Source: CAD feature listing. Evaluate the final solid. Frame: model axes, mm. Face numbers are marked on the shaded views. Coordinates: 2 decimals unless noted, no trailing zeros. Order: outer loops, then holes, each group sorted by start corner. A loop starts at its lowest first (then second) coordinate and runs counter-clockwise, first axis right, second up. Notation, with made-up numbers: (35, 71) -> (71, 71) arc R33 ccw to (71, 109) -> close; hole circle Ø10 at (84.25, -11.5). An arc over 180 degrees is marked (long way). Write item = value, one per line. Start each with the question number.
Item 1: Mould query, pull axis Z, two halves, no side actions, for the marked faces 1, 2 and 3. Classes: released by +Z, released by -Z, zero draft, split by the parting line, or undercut.
Item 2: Contact query for a flat-ended pin moving along its axis: pin 1 (1.9 mm diameter, centred on y = 6.35, z = 0, fed in from +X). Output: stop coordinate, or through.
Item 3: Section query A-A (x = -4). Count the separate pieces of the cut face and the enclosed holes in it, then the cut area to 3 significant figures.
Item 4: Section query B-B (y = 19.05). Output: boundary loops of the cut face in (x, z).
Item 5: Ray query, line 1 along Z through (x, y) = (-5.5, 19.05); line 2 along Y through (x, z) = (-1.25, 2.75) (3 decimals); line 3 along Y through (x, z) = (-8.25, -1) (3 decimals). Return the intervals inside material, ascending. Write a range as [from, to].
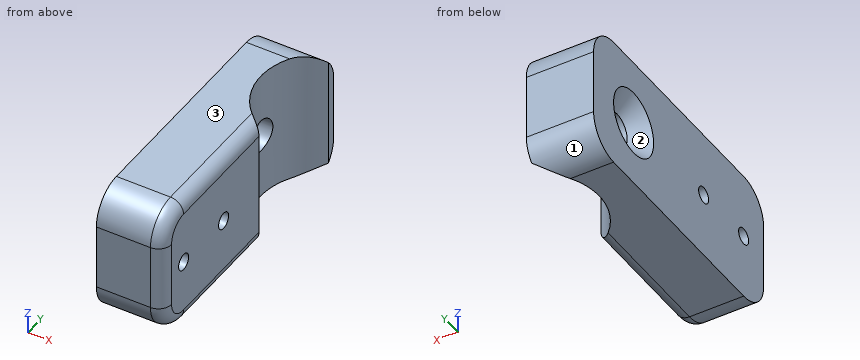
```python
from build123d import *

# Parameters (mm, degrees)
F0_R        = 1.5875
F0_R_2      = 3.175
F1_DEPTH    = 13
F3_DEPTH    = 37.5
F4_T1_DEPTH = 44.75
F5_R        = 2.54
F6_SIZE     = 3.175


# Not quite as in the source:
# - a fillet or chamfer that OpenCascade refuses, or shapes differently, is made with other operations: its cross-section is extruded or revolved along the edge and cut away or added
# - a feature names something its author has since deleted; it is built from what else it names


with BuildPart() as f1:
    # F0 (on Right) → F1 (new body)
    with BuildSketch(Plane.YZ):
        Polygon((0, 0), (0, -12.7), (53.975, -12.7), (53.975, 12.7), (0, 12.7), align=None)
        with Locations((6.35, 0)):
            Circle(F0_R, mode=Mode.SUBTRACT)
        with Locations((19.05, 0)):
            Circle(F0_R, mode=Mode.SUBTRACT)
        with Locations((41.275, 0)):
            Circle(F0_R_2, mode=Mode.SUBTRACT)
    extrude(amount=-F1_DEPTH)

    # F2 (on Top) → F3 (cut, symmetric)
    with BuildSketch(Plane.XY):
        with BuildLine():
            Line((0, 30.2764773719), (0, 52.2735226281))
            ThreePointArc((0, 52.2735226281), (-6.35, 41.275), (0, 30.2764773719))
        make_face()
    extrude(amount=F3_DEPTH, both=True, mode=Mode.SUBTRACT)

    # F4: fillet of radius 6.35 on 4 edges, made by hand

    # F4_s2 → F4_t1 (cut)
    with BuildSketch(Plane.YZ.offset(-28.875)):
        with BuildLine():
            ThreePointArc((0, -6.35), (1.8598719395, -10.8401280605), (6.35, -12.7))
            Line((6.35, -12.7), (0, -12.7))
            Line((0, -12.7), (0, -6.35))
        make_face()
        with BuildLine():
            ThreePointArc((0, 6.35), (1.8598719395, 10.8401280605), (6.35, 12.7))
            Line((6.35, 12.7), (0, 12.7))
            Line((0, 12.7), (0, 6.35))
        make_face()
        with BuildLine():
            ThreePointArc((47.625, -12.7), (52.1151280605, -10.8401280605), (53.975, -6.35))
            Line((53.975, -6.35), (53.975, -12.7))
            Line((53.975, -12.7), (47.625, -12.7))
        make_face()
        with BuildLine():
            ThreePointArc((47.625, 12.7), (52.1151280605, 10.8401280605), (53.975, 6.35))
            Line((53.975, 6.35), (53.975, 12.7))
            Line((53.975, 12.7), (47.625, 12.7))
        make_face()
    extrude(amount=F4_T1_DEPTH, mode=Mode.SUBTRACT)

    # F5
    f5_edges = [f1.edges().sort_by_distance(p)[0] for p in [
        (-6.5, 0, 6.35),
        (0, 0, 0),
        (0, 1.859872, -10.840128),
        (0, 1.859872, 10.840128),
        (0, 18.313239, 12.7),
        (0, 18.313239, -12.7),
    ]]
    fillet(f5_edges, radius=F5_R)

    # F6
    f6_edges = [f1.edges().sort_by_distance(p)[0] for p in [
        (-13, 38.1, 0),
    ]]
    chamfer(f6_edges, length=F6_SIZE)


solid = f1.part
```
Computed:
q1.face_1 = released by -Z
q1.face_2 = undercut
q1.face_3 = released by +Z
q2.pin_1 = through
q3.separate_pieces = 2
q3.enclosed_holes = 2
q3.area = 947 mm^2
q4.outline = (-13, -12.7) -> (-2.54, -12.7) arc R2.54 ccw to (0, -10.16) -> (0, -1.59) -> (-13, -1.59) -> close; (-13, 1.59) -> (0, 1.59) -> (0, 10.16) arc R2.54 ccw to (-2.54, 12.7) -> (-13, 12.7) -> close
q5.line_1 = [-12.7, -1.59], [1.59, 12.7]
q5.line_2 = [0.352, 31.1], [51.45, 53.975]
q5.line_3 = [0, 5.117], [7.583, 17.817], [20.283, 38.262], [44.288, 53.975]
